Part model, mm, in its own coordinate system. Face numbers are marked on the shaded views. A direction names the side the tool comes from. Coordinates: 2 decimals unless noted, no trailing zeros. Order: outer loops, then holes, each group sorted by start corner. A loop starts at its lowest first (then second) coordinate and runs counter-clockwise, first axis right, second up. Notation, with made-up numbers: M -26,-16.5 L 29,-16.5 A23 cw 29,17.5 Z; hole C 72,64 d11. An arc over 180 degrees is marked long. Answer in a Markdown table with one row per item. Add a question column.
from build123d import *

# Parameters (mm, degrees)
F0_R     = 5.08
F1_DEPTH = 50.8
F2_R     = 6.35
F3_DEPTH = 3.175
F4_R     = 6.35
F5_DEPTH = 3.175


with BuildPart() as f1:
    # F0 (on Front) → F1 (new body, symmetric)
    with BuildSketch(Plane.XZ):
        Circle(F0_R)
    extrude(amount=F1_DEPTH, both=True)

    # F2 (on face) → F3 (join)
    with BuildSketch(Plane.XZ.offset(50.8)):
        Circle(F2_R)
    extrude(amount=F3_DEPTH)

    # F4 (on face) → F5 (join)
    with BuildSketch(Plane(origin=(0, 50.8, 0), x_dir=(-1, 0, 0), z_dir=(0, 1, 0))):
        Circle(F4_R)
    extrude(amount=F5_DEPTH)


solid = f1.part
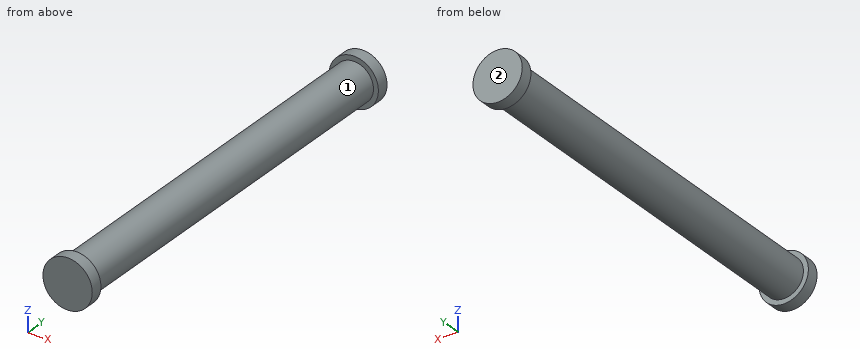
(1) Wall check: line 1 (Y direction, x = 3, z = -4.75) (3 decimals); line 2 (X direction, y = 40.5, z = -1.25); line 3 (X direction, y = 12, z = -3). Give the ranges that are in metal, low to high.
(2) Drop flat-ended pins along their axis: P1, Ø3, axis at x = -4.5, y = -17, coming from the -Z side; P2, Ø5, axis at y = -5.5, z = -4.5, coming from the -X side; P3, Ø1.5, axis at y = -20, z = 2.5, coming from the +X side. Give the stop position or say it passes through.
(3) Slice it at C-C (y = 10.5). List the corners of the cut face in (x, z).
(4) 3-axis set-ups, long thin cutter, end or side, ignore diameter. For the marked faces 1 and 2: which of +Z, -Z, +X, -X, +Y, -Y reach the whole face in a straight line?
(5) Slice it at A-A (x = 0). List the corners of the cut face in (y, z) (3 decimals).
(6) Slice it at B-B (z = 0). List the corners of the cut face in (x, y) (3 decimals), and give its area (3 significant figures).
Computed:
| question | item | result |
|---|---|---|
| 1 | line 1 | y = -53.975 to -50.8, 50.8 to 53.975 |
| 1 | line 2 | x = -4.92 to 4.92 |
| 1 | line 3 | x = -4.1 to 4.1 |
| 2 | P1 | stops at z = -4.1 |
| 2 | P2 | stops at x = -4.67 |
| 2 | P3 | stops at x = 4.77 |
| 3 | outline | C 0,0 d10.16 |
| 4 | face 1 | none |
| 4 | face 2 | +Z, -Z, +X, -X, +Y |
| 5 | outline | M -53.975,-6.35 L -50.8,-6.35 L -50.8,-5.08 L 50.8,-5.08 L 50.8,-6.35 L 53.975,-6.35 L 53.975,6.35 L 50.8,6.35 L 50.8,5.08 L -50.8,5.08 L -50.8,6.35 L -53.975,6.35 Z |
| 6 | outline | M -6.35,-53.975 L 6.35,-53.975 L 6.35,-50.8 L 5.08,-50.8 L 5.08,50.8 L 6.35,50.8 L 6.35,53.975 L -6.35,53.975 L -6.35,50.8 L -5.08,50.8 L -5.08,-50.8 L -6.35,-50.8 Z |
| 6 | area | 1,110 mm^2 |
